```python
from build123d import *
from build123d.topology import SkipClean

# Parameters (mm, degrees)
EXTRUDE_1_DEPTH          = 2.5
REVOLVE_1_ANGLE          = 70
EXTRUDE_2_DEPTH          = 20
EXTRUDE_2_DEPTH_BACK     = 20
SKETCH_4_R               = 2.5
SKETCH_4_R_2             = 1
CUT_EXTRUDE_1_DEPTH      = 18.25
CUT_EXTRUDE_1_DEPTH_BACK = 18.25
SKETCH_5_R               = 1
CUT_EXTRUDE_START        = -100
SKETCH_6_R               = 1
CUT_EXTRUDE_2_DEPTH      = 100
SKETCH_11_R              = 2.5
SKETCH_11_R_2            = 1
EXTRUDE_5_DEPTH          = 1
SKETCH_12_R              = 1
EXTRUDE_6_DEPTH          = 5
SKETCH_13_R              = 1
CUT_EXTRUDE_4_DEPTH      = 10
EXTRUDE_START            = 1
SKETCH_14_R              = 2.5
SKETCH_14_R_2            = 1
EXTRUDE_7_DEPTH          = 1
SKETCH_18_W              = 1.966978086
SKETCH_18_H              = 0.907918652
CUT_EXTRUDE_7_DEPTH      = 10
SKETCH_19_R              = 4.431520752
SKETCH_19_R_2            = 1
CUT_EXTRUDE_8_DEPTH      = 1.75


with BuildPart() as part:
    # Sketch 1 → Extrude 1 (new body)
    with BuildSketch(Plane.XY):
        with BuildLine():
            Line((-20, 0), (-16.5, 0))
            ThreePointArc((-16.5, 0), (0, -16.5), (16.5, 0))
            Line((16.5, 0), (20, 0))
            ThreePointArc((20, 0), (0, -20), (-20, 0))
        make_face()
    extrude(amount=EXTRUDE_1_DEPTH)

    # Sketch 2 → Revolve 1 (revolve)
    with BuildSketch(Plane(origin=(0, 0, 0), x_dir=(-1, 0, 0), z_dir=(0, 0, -1))):
        with BuildLine():
            Line((-18.25, 0), (-16.5, 0))
            ThreePointArc((-16.5, 0), (0, -16.5), (16.5, 0))
            Line((16.5, 0), (18.25, 0))
            ThreePointArc((18.25, 0), (0, -18.25), (-18.25, 0))
        make_face()
    revolve(axis=Axis((16.5, 0, 0), (1, 0, 0)), revolution_arc=REVOLVE_1_ANGLE)

    # Sketch 4 → Extrude 2 (add, two sides: drawn at the far end of the back side and taken through both)
    with SkipClean():  # the faces are left unmerged after this step: merging them gives an invalid solid
        with BuildSketch(Plane(origin=(0, 0, 0), x_dir=(0, 0, -1), z_dir=(1, 0, 0)).offset(-EXTRUDE_2_DEPTH_BACK)):
            with Locations(Location((0, 0, 0), (0, 0, 340))):
                Circle(SKETCH_4_R)
            with Locations(Location((0, 0, 0), (0, 0, 340))):
                Circle(SKETCH_4_R_2, mode=Mode.SUBTRACT)
        extrude(amount=EXTRUDE_2_DEPTH + EXTRUDE_2_DEPTH_BACK)

    # Sketch 5 → Cut-Extrude 1 (cut, two sides: drawn at the far end of the back side and taken through both)
    with SkipClean():  # the faces are left unmerged after this step: merging them gives an invalid solid
        with BuildSketch(Plane(origin=(0, 0, 0), x_dir=(0, 0, -1), z_dir=(1, 0, 0)).offset(-CUT_EXTRUDE_1_DEPTH_BACK)):
            with BuildLine():
                Line((0, -2.5), (-2.5, -2.5))
                Line((-2.5, -2.5), (-2.5, 0))
                ThreePointArc((-2.5, 0), (1.767766953, 1.767766953), (0, -2.5))
            make_face()
            Circle(SKETCH_5_R, mode=Mode.SUBTRACT)
        extrude(amount=CUT_EXTRUDE_1_DEPTH + CUT_EXTRUDE_1_DEPTH_BACK, mode=Mode.SUBTRACT)

    # Sketch 6 → Cut-Extrude 2 (cut)
    with SkipClean():  # the faces are left unmerged after this step: merging them gives an invalid solid
        with BuildSketch(Plane(origin=(20, 0, 0), x_dir=(0, 0, -1), z_dir=(1, 0, 0)).offset(CUT_EXTRUDE_START)):
            Circle(SKETCH_6_R)
        extrude(amount=CUT_EXTRUDE_2_DEPTH, mode=Mode.SUBTRACT)

    # Sketch 11 → Extrude 5 (add)
    with SkipClean():  # the faces are left unmerged after this step: merging them gives an invalid solid
        with BuildSketch(Plane(origin=(20, 0, 0), x_dir=(0, 0, -1), z_dir=(1, 0, 0))):
            Circle(SKETCH_11_R)
            Circle(SKETCH_11_R_2, mode=Mode.SUBTRACT)
        extrude(amount=EXTRUDE_5_DEPTH)

    # Sketch 12 → Extrude 6 (add)
    with BuildSketch(Plane.ZY.offset(20)):
        with BuildLine():
            ThreePointArc((2.494892647, -0.15972063), (0.003121638, -2.499998051), (-2.494485996, -0.165950649))
            Line((-2.494485996, -0.165950649), (-2.494485996, -8.665950649))
            Line((-2.494485996, -8.665950649), (2.505514004, -8.665950649))
            Line((2.505514004, -8.665950649), (2.494892647, -0.15972063))
        make_face()
        with Locations((0, -7)):
            Circle(SKETCH_12_R, mode=Mode.SUBTRACT)
    extrude(amount=-EXTRUDE_6_DEPTH)

    # Sketch 13 → Cut-Extrude 4 (cut)
    with BuildSketch(Plane.ZY.offset(20)):
        with Locations((0, -7)):
            Circle(SKETCH_13_R)
    extrude(amount=-CUT_EXTRUDE_4_DEPTH, mode=Mode.SUBTRACT)

    # Sketch 14 → Extrude 7 (add)
    with BuildSketch(Plane.ZY.offset(20).offset(EXTRUDE_START)):
        with Locations(Location((0, 0, 0), (0, 0, 180))):
            Circle(SKETCH_14_R)
        with Locations(Location((0, 0, 0), (0, 0, 180))):
            Circle(SKETCH_14_R_2, mode=Mode.SUBTRACT)
    extrude(amount=-EXTRUDE_7_DEPTH)

    # Sketch 16 → Cut-Revolve 1 (revolve, cut)
    with BuildSketch(Plane.XY):
        with BuildLine():
            Line((16.5, 0), (-16.5, 0))
            ThreePointArc((-16.5, 0), (0, -16.5), (16.5, 0))
        make_face()
    revolve(axis=Axis((0, 0, 0), (1, 0, 0)), mode=Mode.SUBTRACT)

    # Sketch 18 → Cut-Extrude 7 (cut)
    with SkipClean():  # the faces are left unmerged after this step: merging them gives an invalid solid
        with BuildSketch(Plane(origin=(0, 0, -2.494485996), x_dir=(-1, 0, 0), z_dir=(0, 0, -1))):
            with Locations((17.268550398, -0.453959326)):
                Rectangle(SKETCH_18_W, SKETCH_18_H)
        extrude(amount=-CUT_EXTRUDE_7_DEPTH, mode=Mode.SUBTRACT)
    add(part.part.scale(1), mode=Mode.REPLACE)  # the faces are merged on a copy

    # Sketch 19 → Cut-Extrude 8 (cut)
    with BuildSketch(Plane.ZY.offset(20)):
        with Locations((0, -7)):
            Circle(SKETCH_19_R)
        with Locations((0, -7)):
            Circle(SKETCH_19_R_2, mode=Mode.SUBTRACT)
    extrude(amount=-CUT_EXTRUDE_8_DEPTH, mode=Mode.SUBTRACT)


solid = part.part
```
For this review, take the finished solid that the model builds, in its own axes (mm). A direction names the side the tool comes from. Round coordinates to 2 decimals unless told otherwise and drop trailing zeros. Write each loop counter-clockwise with the first axis right and the second up, starting at its lowest first coordinate (ties: lowest second). Pieces come first, ordered by that corner, then holes. Notation, with made-up numbers: (13.5, 17.5) - (24.5, 17.5) arc R26 cw to (24.5, 52.5) - close; hole circle Ø9 at (-38.75, 52.5). An arc over 180 degrees is marked (long way). Put each result on its own line as item: value.
Q1. Insertion check: pin 1 Ø1.2 at (y, z) = (-7.5, 1.5) entering from +X; pin 2 Ø3 at (x, y) = (-18, -1.5) entering from +Z; pin 3 Ø1.6 at (y, z) = (0, 0) entering from +X; pin 4 Ø8 at (y, z) = (-11, -4.5) entering from -X. Each pin has a flat end and moves straight along its axis. Give the tip position at first contact, or say it passes through.
Solved:
pin 1: stops at x = 18.77
pin 2: stops at z = 2.5
pin 3: passes through
pin 4: stops at x = -18.25
Q2. We need section B-B (y = -16). Give the boundary of the cut face in (x, z), and give its area (3 significant figures).
Solved:
outline: (-12, 0) - (-8.78, 0) arc R8.78 ccw to (8.78, 0) - (12, 0) - (12, 2.5) - (4.03, 2.5) - (4.03, 0) arc R4.03 cw to (-4.03, 0) - (-4.03, 2.5) - (-12, 2.5) - close
area: 135 mm2
Q3. We need section A-A (x = 5). Give the boundary of the cut face in (y, z), and give its area (4 significant figures).
Solved:
outline: (-19.36, 0) - (-17.55, 0) arc R17.55 ccw to (-6, -16.49) - (-5.38, -14.78) arc R15.72 cw to (-15.72, 0) - (-15.72, 2.5) - (-19.36, 2.5) - close
area: 46.25 mm2
Q4. Machinability: for faces 4 (the face through (-16, -8, 0)), 5 (the face through (-18, -4, -2.494)), 6 (the face through (-18.25, -2, 0)), 7 (the face through (18.25, -1, 1)), which of the approach directions +Z, -Z, +X, -X, +Y, -Y give a long, thin tool a straight path to every point of the face, cutting with its end or side? Answer none if there is none.
Solved:
face 4: -X
face 5: -Z, -X, -Y
face 6: +Y
face 7: +Z, -Z, +Y
Q5. Wall thickness on probe 1 along Y at (x, z) = (20.2, 0); probe 2 along X at (y, z) = (-1.75, 0.25): over which ranges is each line inside the solid? List them lowest first.
Solved:
probe 1: y = -2.5 to -1, 1 to 2.5
probe 2: x = -21 to -18.25, 18.25 to 21
Q6. We need section D-D (x = 0.5). Give the boundary of the cut face in (y, z), and give its area (3 significant figures).
Solved:
outline: (-19.99, 0) - (-18.24, 0) arc R18.24 ccw to (-6.24, -17.14) - (-5.64, -15.5) arc R16.49 cw to (-16.49, 0) - (-16.49, 2.5) - (-19.99, 2.5) - close
area: 45.9 mm2
Q7. Mouldability with a two-part tool opening along X and no side actions: class faces 1 (the face through (-19.14, -2.57, 0.04)), 2 (the face through (17, -2.5, 1)), 3 (the face through (-21, 1, -1)) as released by +X, released by -X, zero draft, split by the parting line, or undercut.
Solved:
face 1: zero draft
face 2: undercut
face 3: released by -X
